Here's how the part is built. I have some questions about the finished solid (model axes, mm). A direction names the side the tool comes from. Coordinates: 2 decimals unless noted, no trailing zeros. Write each loop counter-clockwise with the first axis right and the second up, starting at its lowest first coordinate (ties: lowest second). Pieces come first, ordered by that corner, then holes.
```python
from build123d import *

# Parameters (mm, degrees)
BOSS_EXTRUDE1_DEPTH      = 286
BOSS_EXTRUDE1_DEPTH_BACK = 286
SKETCH1_W                = 20
SKETCH1_H                = 20
SKETCH1_W_2              = 17.6
SKETCH1_H_2              = 17.6
SKETCH2_W                = 36
SKETCH2_H                = 20
BOSS_EXTRUDE2_DEPTH      = 3
SKETCH3_R                = 3
CUT_EXTRUDE1_DEPTH       = 308.748273756
BOSS_EXTRUDE3_DEPTH      = 10
SKETCH5_R                = 2
BOSS_EXTRUDE4_DEPTH      = 10
CHAMFER1_SIZE            = 0.5
SKETCH6_W                = 36
SKETCH6_H                = 20
BOSS_EXTRUDE5_DEPTH      = 3
CHAMFER2_SIZE            = 0.5
SKETCH7_W                = 3
SKETCH7_H                = 20
BOSS_EXTRUDE6_DEPTH      = 2
SKETCH8_W                = 3
SKETCH8_H                = 6
CUT_EXTRUDE2_DEPTH       = 5
BOSS_EXTRUDE7_DEPTH      = 2
BOSS_EXTRUDE7_DEPTH_BACK = 25
SKETCH9_R                = 3


with BuildPart() as part:
    # Sketch1 → Boss-Extrude1 (new, two sides: drawn at the far end of the back side and taken through both)
    with BuildSketch(Plane.XY.offset(-BOSS_EXTRUDE1_DEPTH_BACK)):
        with Locations((0, -92)):
            Rectangle(SKETCH1_W, SKETCH1_H)
        with Locations((0, -92)):
            Rectangle(SKETCH1_W_2, SKETCH1_H_2, mode=Mode.SUBTRACT)
    extrude(amount=BOSS_EXTRUDE1_DEPTH + BOSS_EXTRUDE1_DEPTH_BACK)

    # Sketch2 → Boss-Extrude2 (add)
    with BuildSketch(Plane(origin=(0, 0, -286), x_dir=(-1, 0, 0), z_dir=(0, 0, -1))):
        with Locations((0, -92)):
            Rectangle(SKETCH2_W, SKETCH2_H)
    extrude(amount=BOSS_EXTRUDE2_DEPTH)

    # Sketch3 → Cut-Extrude1 (cut, through all)
    with BuildSketch(Plane(origin=(10, 0, 0), x_dir=(0, 0, -1), z_dir=(1, 0, 0))):
        with Locations((-106, -92)):
            Circle(SKETCH3_R)
        with Locations((-94, -92)):
            Circle(SKETCH3_R)
        with Locations((94, -92)):
            Circle(SKETCH3_R)
        with Locations((106, -92)):
            Circle(SKETCH3_R)
    extrude(amount=-CUT_EXTRUDE1_DEPTH, mode=Mode.SUBTRACT)

    # Sketch4 → Boss-Extrude3 (add)
    with BuildSketch(Plane(origin=(0, -82, 0), x_dir=(1, 0, 0), z_dir=(0, 1, 0))):
        with BuildLine():
            Line((18, 286), (19.722941986, 285.711382236))
            ThreePointArc((19.722941986, 285.711382236), (25.543178803, 290.856309234), (18, 289))
            Line((18, 289), (18, 286))
        make_face()
    boss_extrude3 = extrude(amount=-BOSS_EXTRUDE3_DEPTH)

    # Sketch5 → Boss-Extrude4 (add)
    with BuildSketch(Plane.XZ.offset(92)):
        with Locations(Location((22, -289, 0), (0, 0, 90))):
            Circle(SKETCH5_R)
    boss_extrude4 = extrude(amount=BOSS_EXTRUDE4_DEPTH)

    # Chamfer1
    chamfer1_edges = [part.edges().sort_by_distance(p)[0] for p in [
        (22, -102, -291),
    ]]
    chamfer(chamfer1_edges, length=CHAMFER1_SIZE)

    # Sketch6 → Boss-Extrude5 (add)
    with BuildSketch(Plane.XY.offset(286)):
        with Locations((0, -92)):
            Rectangle(SKETCH6_W, SKETCH6_H)
    extrude(amount=BOSS_EXTRUDE5_DEPTH)

    # Mirror5: Boss-Extrude3, Boss-Extrude4 across plane
    add(boss_extrude3.mirror(Plane.XY))
    add(boss_extrude4.mirror(Plane.XY))

    # Chamfer2
    chamfer2_edges = [part.edges().sort_by_distance(p)[0] for p in [
        (22, -102, 291),
    ]]
    chamfer(chamfer2_edges, length=CHAMFER2_SIZE)

    # Sketch7 → Boss-Extrude6 (add)
    with BuildSketch(Plane.ZY.offset(18)):
        with Locations((287.5, -92)):
            Rectangle(SKETCH7_W, SKETCH7_H)
    boss_extrude6 = extrude(amount=BOSS_EXTRUDE6_DEPTH)

    # Sketch8 → Cut-Extrude2 (cut)
    with BuildSketch(Plane.ZY.offset(20)):
        with Locations((287.5, -92)):
            Rectangle(SKETCH8_W, SKETCH8_H)
    cut_extrude2 = extrude(amount=-CUT_EXTRUDE2_DEPTH, mode=Mode.SUBTRACT)

    # Mirror6: Boss-Extrude6, Cut-Extrude2 across plane
    add(boss_extrude6.mirror(Plane.XY))
    add(cut_extrude2.mirror(Plane.XY), mode=Mode.SUBTRACT)

    # Sketch9 → Boss-Extrude7 (add, two sides: drawn at the far end of the back side and taken through both)
    with BuildSketch(Plane.ZY.offset(10).offset(-BOSS_EXTRUDE7_DEPTH_BACK)):
        with Locations(Location((94, -92, 0), (0, 0, 90))):
            Circle(SKETCH9_R)
        with Locations(Location((-94, -92, 0), (0, 0, 90))):
            Circle(SKETCH9_R)
    extrude(amount=BOSS_EXTRUDE7_DEPTH + BOSS_EXTRUDE7_DEPTH_BACK)


solid = part.part
```
1) Will these pins go through, and if not, where does the flat tip stop? pin 1 (1.8 mm diameter, centred on y = -91, z = -94, fed in from +X); pin 2 (6 mm diameter, centred on y = -96.5, z = 3, fed in from -X); pin 3 (3 mm diameter, centred on y = -92, z = -94.5, fed in from -X).
Values follow:
pin 1: stops at x = 15
pin 2: stops at x = -10
pin 3: stops at x = -12
2) We'd pull the mould along X, two halves only. Please class faces 1 (the face through (-2, -82, 4)), 2 (the face through (-10, -92, -4)), 3 (the face through (-8.8, -92, -4)): pulls with the +X half, pulls with the -X half, needs draft (parallel to the pull), parting line crosses it, or undercut.
Values follow:
face 1: needs draft
face 2: pulls with the -X half
face 3: undercut
3) I need wall thicknesses on probe 1 along Z at (x, y) = (6.5, -83.75); probe 2 along Y at (x, z) = (-9, 106); probe 3 along X at (y, z) = (-86.75, -105.5). Which ranges of each line are inside material? Lowest first, please.
Values follow:
probe 1: z = -289 to -286, 286 to 289
probe 2: y = -102 to -95, -89 to -82
probe 3: x = -10 to -8.8, 8.8 to 10
4) Imagine slicing it at A-A on x = -2.5. Please give me the cut outline in (y, z).
Values follow:
outline: (-102, -289) - (-82, -289) - (-82, 289) - (-102, 289) - close; circle Ø6 at (-92, -94); circle Ø6 at (-92, 94); hole (-100.8, -286) - (-83.2, -286) - (-83.2, 286) - (-100.8, 286) - close
5) On a 3-axis mill with a long thin cutter (end or side, diameter ignored), from which of +Z, -Z, +X, -X, +Y, -Y can I reach the whole of each face in a straight line? I mean faces 4 (the face through (0, -92, -286)), 5 (the face through (-1, -92, -289)), 6 (the face through (-1, -102, 4)), 7 (the face through (-14, -92, 286)), 8 (the face through (-1, -92, 289)). Say none if no direction works.
Values follow:
face 4: none
face 5: -Z, -X, +Y, -Y
face 6: +Z, -Z, +X, -X, -Y
face 7: -X, +Y, -Y
face 8: +Z, -X, +Y, -Y
6) Imagine slicing it at B-B on z = 73.5. Please give me the cut outline in (x, y), then the cut area to 3 significant figures.
Values follow:
outline: (-10, -102) - (10, -102) - (10, -82) - (-10, -82) - close; hole (-8.8, -100.8) - (8.8, -100.8) - (8.8, -83.2) - (-8.8, -83.2) - close
area: 90.2 mm2
